Work out the finished part from the listing and answer in its coordinate system (mm). Coordinates: 2 decimals unless noted, no trailing zeros. Write each loop counter-clockwise with the first axis right and the second up, starting at its lowest first coordinate (ties: lowest second). Pieces come first, ordered by that corner, then holes. Notation, with made-up numbers: (75.5, -0.5) - (99.5, -0.5) arc R25 cw to (99.5, 24.5) - close; hole circle Ø5 at (87, 45). An arc over 180 degrees is marked (long way). Use one line per item in the form item = value. Start each with the question number.
Item 1: A cutting plane is placed at A-A (x = 5). Write down the section's boundary in (y, z) (3 decimals).
Item 2: Given pin 1 (3 mm diameter, centred on y = 15, z = 362.425, fed in from -X), flat-ended and moving along its own axis, determine where the tip first touches the part or whether it passes through.
Item 3: Consider probe 1 along Z at (x, y) = (6.5, 22.75); probe 2 along Z at (x, y) = (4, 9.75); probe 3 along X at (y, z) = (9.5, 12). Determine where each line is inside the solid, lowest interval first.
from build123d import *

# Parameters (mm, degrees)
SKETCH1_W               = 10
SKETCH1_H               = 30
BOSS_EXTRUDE1_DEPTH     = 440
ESQUISSE1_R             = 1.65
ENL_V_MAT_EXTRU_1_DEPTH = 442.134900002
ESQUISSE2_R             = 2
ENL_V_MAT_EXTRU_2_DEPTH = 442.134900002


with BuildPart() as part:
    # Sketch1 → Boss-Extrude1 (new body)
    with BuildSketch(Plane.XY):
        with Locations((5, 15)):
            Rectangle(SKETCH1_W, SKETCH1_H)
    extrude(amount=BOSS_EXTRUDE1_DEPTH)

    # Esquisse1 → Enlèv. mat.-Extru.1 (cut, through all)
    with BuildSketch(Plane(origin=(0, 30, 0), x_dir=(1, 0, 0), z_dir=(0, 1, 0))):
        with Locations(Location((5, -428, 0), (0, 0, 270))):
            Circle(ESQUISSE1_R)
        with Locations(Location((5, -12, 0), (0, 0, 270))):
            Circle(ESQUISSE1_R)
    extrude(amount=-ENL_V_MAT_EXTRU_1_DEPTH, mode=Mode.SUBTRACT)

    # Esquisse2 → Enlèv. mat.-Extru.2 (cut, through all)
    with BuildSketch(Plane(origin=(10, 0, 0), x_dir=(0, 0, -1), z_dir=(1, 0, 0))):
        with Locations((-362.425, 15)):
            Circle(ESQUISSE2_R)
        with Locations((-77.575, 15)):
            Circle(ESQUISSE2_R)
        with Locations((-322.04, 15)):
            Circle(ESQUISSE2_R)
        with Locations((-117.96, 15)):
            Circle(ESQUISSE2_R)
    extrude(amount=-ENL_V_MAT_EXTRU_2_DEPTH, mode=Mode.SUBTRACT)


solid = part.part
Answer:
q1.outline = (0, 0) - (30, 0) - (30, 10.35) - (0, 10.35) - close; (0, 13.65) - (30, 13.65) - (30, 426.35) - (0, 426.35) - close; (0, 429.65) - (30, 429.65) - (30, 440) - (0, 440) - close; hole circle Ø4 at (15, 77.575); hole circle Ø4 at (15, 117.96); hole circle Ø4 at (15, 322.04); hole circle Ø4 at (15, 362.425)
q2.pin_1 = through
q3.probe_1 = 0 to 11.31, 12.69 to 427.31, 428.69 to 440
q3.probe_2 = 0 to 10.69, 13.31 to 426.69, 429.31 to 440
q3.probe_3 = 0 to 3.35, 6.65 to 10
